from build123d import *

# Parameters (mm, degrees)
BOSS_EXTRUDE1_DEPTH = 6.35


with BuildPart() as part:
    # Sketch1 → Boss-Extrude1 (new body)
    with BuildSketch(Plane(origin=(0, 0, 0), x_dir=(1, 0, 0), z_dir=(0, 1, 0))):
        with BuildLine():
            ThreePointArc((-3.81, 3.81), (-2.694076836, 1.115923164), (0, 0))
            Line((0, 0), (0, 7.62))
            ThreePointArc((0, 7.62), (-2.387181834, 6.779421306), (-3.721022887, 4.628589444))
            Line((-3.721022887, 4.628589444), (-3.81, 3.81))
        make_face()
        with BuildLine():
            ThreePointArc((-3.721022887, 4.628589444), (-2.387181834, 6.779421306), (0, 7.62))
            Line((0, 7.62), (0, 38.862))
            Line((0, 38.862), (-3.721022887, 4.628589444))
        make_face()
        with BuildLine():
            Line((0, 7.62), (0, 0))
            ThreePointArc((0, 0), (2.694076836, 1.115923164), (3.81, 3.81))
            Line((3.81, 3.81), (3.721022887, 4.628589444))
            ThreePointArc((3.721022887, 4.628589444), (2.387181834, 6.779421306), (0, 7.62))
        make_face()
        with BuildLine():
            Line((0, 38.862), (0, 7.62))
            ThreePointArc((0, 7.62), (2.387181834, 6.779421306), (3.721022887, 4.628589444))
            Line((3.721022887, 4.628589444), (0, 38.862))
        make_face()
    extrude(amount=BOSS_EXTRUDE1_DEPTH)


solid = part.part
Check sheet for the modelled part. Datum: model origin and axes. Units: mm. Give positions to 0.01 mm unless a question says otherwise; leave off trailing zeros. Write each loop counter-clockwise with the first axis right and the second up, starting at its lowest first coordinate (ties: lowest second). Pieces come first, ordered by that corner, then holes. Notation, with made-up numbers: (-5.5, -15.75) -> (37.5, -15.75) arc R9 cw to (37.5, -0.75) -> close; hole circle Ø6 at (-15, -24). An arc over 180 degrees is marked (long way). Write item = value, one per line.
Item 1: Scan lines: probe 1 along X at (y, z) = (3.75, -23); probe 2 along X at (y, z) = (1, -37). Record each from-to range of solid material in increasing order. Write a range as from..to.
Output:
probe_1 = -1.72..1.72
probe_2 = -0.2..0.2
Item 2: Sectioned sample at B-B on x = 0.5. Record the boundary of the cut face in (y, z).
Output:
outline = (0, -34.26) -> (6.35, -34.26) -> (6.35, -0.03) -> (0, -0.03) -> close
Item 3: Gauge pin test, flat ends, axial feed: pin 1 (2 mm diameter, centred on x = 0.5, y = 1, fed in from +Z); pin 2 (1.5 mm diameter, centred on x = -2.5, y = 2.5, fed in from +Z). Record the tip position at first contact, or that the pin passes through.
Output:
pin_1 = 0
pin_2 = -0.43
Item 4: Sectioned sample at A-A on y = 3.5. Record the boundary of the cut face in (x, z), and give its area (3 significant figures).
Output:
outline = (-3.81, -3.81) -> (0, -38.86) -> (3.81, -3.81) arc R3.81 ccw to start
area = 156 mm^2
Item 5: Sectioned sample at C-C on z = -24. Record the boundary of the cut face in (x, y).
Output:
outline = (-1.62, 0) -> (1.62, 0) -> (1.62, 6.35) -> (-1.62, 6.35) -> close
